Work out the finished part from the listing and answer in its coordinate system (mm). Face numbers are marked on the shaded views. Round coordinates to 2 decimals unless told otherwise and drop trailing zeros. Write each loop counter-clockwise with the first axis right and the second up, starting at its lowest first coordinate (ties: lowest second). Pieces come first, ordered by that corner, then holes. Notation, with made-up numbers: M 18.25,85 L 31.25,85 A14 ccw 31.25,109 Z; hole C 51.5,-34.75 d5. An arc over 180 degrees is marked long. Answer in a Markdown table with one row per item.
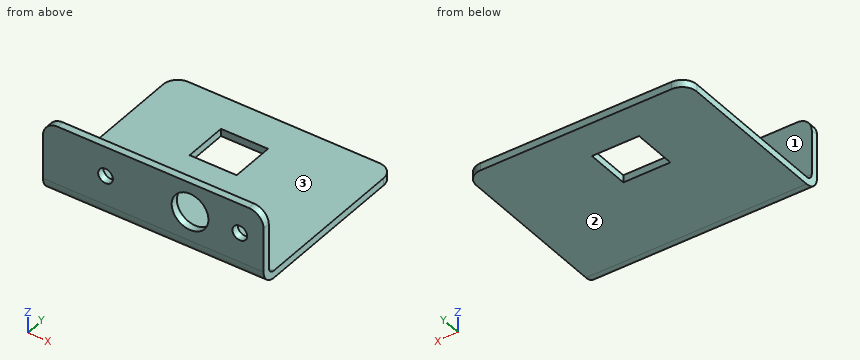
```python
from build123d import *

# Parameters (mm, degrees)
BOSS_EXTRUDE1_DEPTH    = 38.1
SKETCH2_W              = 8.128
SKETCH2_H              = 7.62
CUT_EXTRUDE1_DEPTH     = 52.195336702
CONVERT_SOLID1_DEPTH   = 38.1
CONVERT_SOLID1_2_DEPTH = 38.1
FILLET1_R              = 2.54
SKETCH7_R              = 3.175
CUT_EXTRUDE2_DEPTH     = 52.195336702
SKETCH8_R              = 1.27
CUT_EXTRUDE3_DEPTH     = 52.195336702


# Read off the part's stored shape, not the designer's step: Convert-Solid1
with BuildPart() as part:
    # Sketch1 → Boss-Extrude1 (new body)
    with BuildSketch(Plane(origin=(0, 0, 0), x_dir=(0, 0, -1), z_dir=(1, 0, 0))):
        Polygon((0, 0), (12.7, 0), (12.7, 31.75), (11.43, 31.75), (11.43, 1.27), (0, 1.27), align=None)
    extrude(amount=BOSS_EXTRUDE1_DEPTH)

    # Sketch2 → Cut-Extrude1 (cut, through all)
    with BuildSketch(Plane(origin=(0, 0, -12.7), x_dir=(-1, 0, 0), z_dir=(0, 0, -1))):
        with Locations((-16.764, 21.59)):
            Rectangle(SKETCH2_W, SKETCH2_H)
    extrude(amount=-CUT_EXTRUDE1_DEPTH, mode=Mode.SUBTRACT)

    # Convert-Solid1 outline → Convert-Solid1 (cut)
    with BuildSketch(Plane.YZ):
        with BuildLine():
            ThreePointArc((2.54, -12.7), (0.743948776, -11.956051224), (0, -10.16))
            Line((0, -10.16), (0, -12.7))
            Line((0, -12.7), (2.54, -12.7))
        make_face()
    extrude(amount=CONVERT_SOLID1_DEPTH, mode=Mode.SUBTRACT)

    # Convert-Solid1 2 outline → Convert-Solid1 2 (add)
    with BuildSketch(Plane.YZ):
        with BuildLine():
            ThreePointArc((2.54, -11.43), (1.641974388, -11.058025612), (1.27, -10.16))
            Line((1.27, -10.16), (1.27, -11.43))
            Line((1.27, -11.43), (2.54, -11.43))
        make_face()
    extrude(amount=CONVERT_SOLID1_2_DEPTH)

    # Fillet1
    fillet1_edges = [part.edges().sort_by_distance(p)[0] for p in [
        (0, 31.75, -12.065),
        (38.1, 31.75, -12.065),
        (38.1, 0.635, 0),
        (0, 0.635, 0),
    ]]
    fillet(fillet1_edges, radius=FILLET1_R)

    # Sketch7 → Cut-Extrude2 (cut, through all)
    with BuildSketch(Plane.XZ):
        with Locations(Location((25.4, -5.08, 0), (0, 0, 270))):
            Circle(SKETCH7_R)
    extrude(amount=-CUT_EXTRUDE2_DEPTH, mode=Mode.SUBTRACT)

    # Sketch8 → Cut-Extrude3 (cut, through all)
    with BuildSketch(Plane.XZ):
        with Locations(Location((10.8, -5.08, 0), (0, 0, 270))):
            Circle(SKETCH8_R)
        with Locations(Location((34, -5.08, 0), (0, 0, 270))):
            Circle(SKETCH8_R)
    extrude(amount=-CUT_EXTRUDE3_DEPTH, mode=Mode.SUBTRACT)


solid = part.part
```
1. Given pin 1 (3 mm diameter, centred on x = 17, y = 17, fed in from +Z); pin 2 (4 mm diameter, centred on x = 25.4, z = -5.08, fed in from -Y); pin 3 (3 mm diameter, centred on x = 34, z = -5.08, fed in from +Y); pin 4 (0.6 mm diameter, centred on x = 16.5, z = -12, fed in from -Y), each flat-ended and moving along its own axis, determine where each tip first touches the part or whether it passes through.
Calculated:
| item | result |
|---|---|
| pin 1 | stops at z = -11.43 |
| pin 2 | passes through |
| pin 3 | stops at y = 1.27 |
| pin 4 | stops at y = 0.52 |
2. Determine the mould class of the marked faces 1, 2 and 3 for opening direction Z: released by +Z, released by -Z, zero draft, split by the parting line, or undercut.
Calculated:
| item | result |
|---|---|
| face 1 | zero draft |
| face 2 | released by -Z |
| face 3 | released by +Z |
3. The part is cut by section B-B (y = 24.5). Determine the outline of the cut face in (x, z).
Calculated:
| item | result |
|---|---|
| outline | M 0,-12.7 L 12.7,-12.7 L 12.7,-11.43 L 0,-11.43 Z; M 20.83,-12.7 L 38.1,-12.7 L 38.1,-11.43 L 20.83,-11.43 Z |
4. Consider line 1 along X through (y, z) = (0.95, -5.08) (3 decimals); line 2 along Y through (x, z) = (7.5, -0.75); line 3 along X through (y, z) = (20, -12). Determine where each line is inside the solid, lowest interval first. Write a range as from..to.
Calculated:
| item | result |
|---|---|
| line 1 | x = 0..9.53, 12.07..22.225, 28.575..32.73, 35.27..38.1 |
| line 2 | y = 0..1.27 |
| line 3 | x = 0..12.7, 20.83..38.1 |
5. The part is cut by section D-D (x = 25.4). Determine the outline of the cut face in (y, z) (3 decimals), plus the area to 3 significant figures.
Calculated:
| item | result |
|---|---|
| outline | M 0,-10.16 A2.54 ccw 2.54,-12.7 L 31.75,-12.7 L 31.75,-11.43 L 2.54,-11.43 A1.27 cw 1.27,-10.16 L 1.27,-8.255 L 0,-8.255 Z; M 0,-1.905 L 1.27,-1.905 L 1.27,0 L 0,0 Z |
| area | 45.7 mm² |
6. The part is cut by section C-C (z = -5.08). Determine the outline of the cut face in (x, y) (3 decimals), plus the area to 3 significant figures.
Calculated:
| item | result |
|---|---|
| outline | M 0,0 L 9.53,0 L 9.53,1.27 L 0,1.27 Z; M 12.07,0 L 22.225,0 L 22.225,1.27 L 12.07,1.27 Z; M 28.575,0 L 32.73,0 L 32.73,1.27 L 28.575,1.27 Z; M 35.27,0 L 38.1,0 L 38.1,1.27 L 35.27,1.27 Z |
| area | 33.9 mm² |
7. The part is cut by section A-A (x = 34). Determine the outline of the cut face in (y, z), plus the area to 3 significant figures.
Calculated:
| item | result |
|---|---|
| outline | M 0,-10.16 A2.54 ccw 2.54,-12.7 L 31.75,-12.7 L 31.75,-11.43 L 2.54,-11.43 A1.27 cw 1.27,-10.16 L 1.27,-6.35 L 0,-6.35 Z; M 0,-3.81 L 1.27,-3.81 L 1.27,0 L 0,0 Z |
| area | 50.6 mm² |
